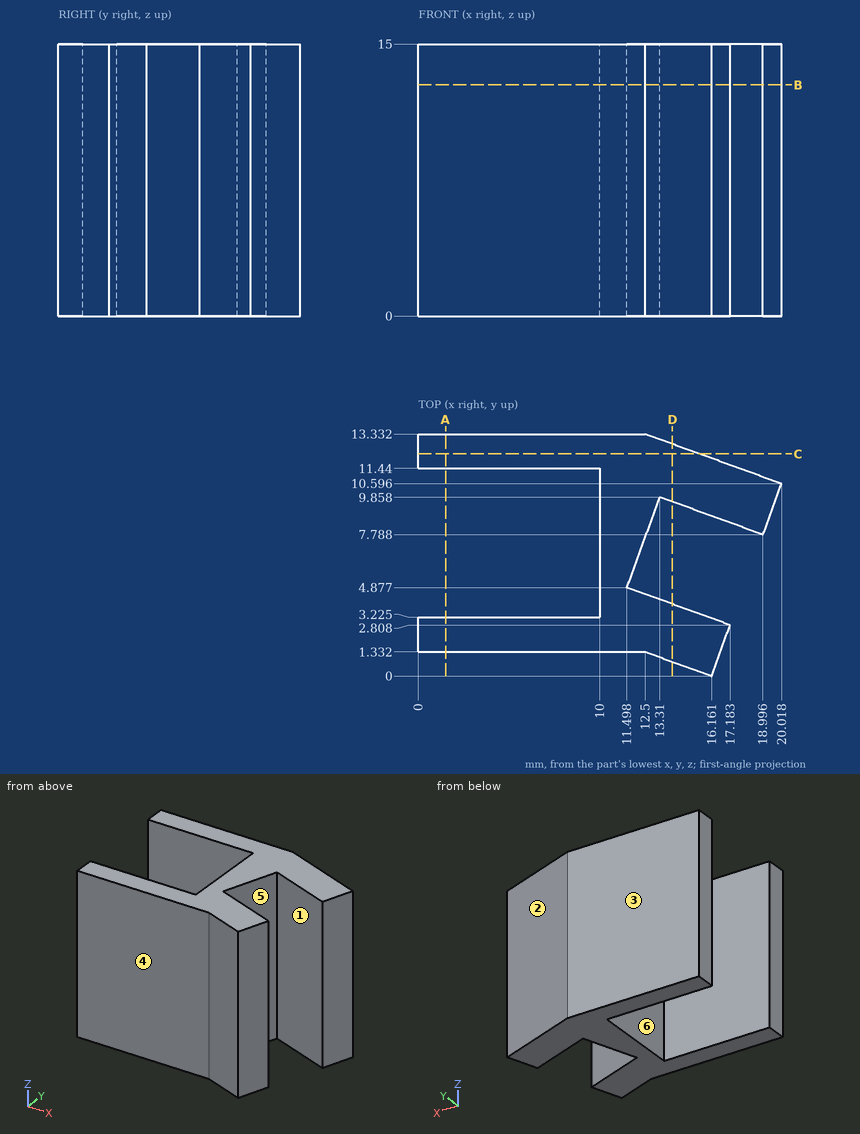
Source: three-view drawing plus pictorial views. Frame: mm from the lowest corner of the part. A direction names the side the tool comes from. Coordinates: 2 decimals unless noted, no trailing zeros. Order: outer loops, then holes, each group sorted by start corner. A loop starts at its lowest first (then second) coordinate and runs counter-clockwise, first axis right, second up. Notation, with made-up numbers: M -38.5,32 L -9.5,32 A29 ccw -9.5,56 Z; hole C -26,41 d2. An arc over 180 degrees is marked long. One line per question, with ' | ' between items.
Item 1: Section A-A (x = 1.5). Output: boundary loops of the cut face in (y, z) (1 decimal).
Geometry results:
outline: M 1.3,0 L 3.2,0 L 3.2,15 L 1.3,15 Z; M 11.4,0 L 13.3,0 L 13.3,15 L 11.4,15 Z
Item 2: Section C-C (y = 12.25). Output: boundary loops of the cut face in (x, z).
Geometry results:
outline: M 0,0 L 15.47,0 L 15.47,15 L 0,15 Z
Item 3: Reachability of the marked faces 4, 5 and 6 from +Z, -Z, +X, -X, +Y, -Y: full face, straight path, thin tool, end or side. Return the list, or none.
Geometry results:
face 4: +Z, -Z, -X, -Y | face 5: +Z, -Z | face 6: +Z, -Z, -X
Item 4: Section D-D (x = 14). Output: boundary loops of the cut face in (y, z).
Geometry results:
outline: M 0.79,0 L 3.97,0 L 3.97,15 L 0.79,15 Z; M 9.61,0 L 12.79,0 L 12.79,15 L 9.61,15 Z
Item 5: Ray query, line 1 along Y through (x, z) = (1.25, 10.5) (1 decimal); line 2 along Y through (x, z) = (10.5, 2.5); line 3 along Y through (x, z) = (16, 5). Return the intervals inside material, ascending.
Geometry results:
line 1: y = 1.3 to 3.2, 11.4 to 13.3 | line 2: y = 1.33 to 13.33 | line 3: y = 0.06 to 3.24, 8.88 to 12.06
Item 6: Draft query along X for the marked faces 1, 2 and 3. Return one class per face: released by +X, released by -X, zero draft, split by the parting line, or undercut.
Geometry results:
face 1: undercut | face 2: released by +X | face 3: zero draft
Item 7: Pin query (flat end, axial travel): pin 1 (8 mm diameter, centred on x = 4.5, z = 10.5, fed in from -Y); pin 2 (4 mm diameter, centred on y = 5.5, z = 10.5, fed in from -X); pin 3 (3 mm diameter, centred on y = 9, z = 5.5, fed in from +X). Return the tip coordinate at first contact, or that it passes through.
Geometry results:
pin 1: stops at y = 1.33 | pin 2: stops at x = 10 | pin 3: stops at x = 19.98
Item 8: Section B-B (z = 12.75). Output: boundary loops of the cut face in (x, y) (1 decimal), then the cut area to 3 significant figures.
Geometry results:
outline: M 0,1.3 L 12.5,1.3 L 16.2,0 L 17.2,2.8 L 11.5,4.9 L 13.3,9.9 L 19,7.8 L 20,10.6 L 12.5,13.3 L 0,13.3 L 0,11.4 L 10,11.4 L 10,3.2 L 0,3.2 Z | area: 103 mm^2
